Check sheet for the modelled part. Datum: model origin and axes. Units: mm. Face numbers are marked on the shaded views. A direction names the side the tool comes from. Coordinates: 2 decimals unless noted, no trailing zeros. Write each loop counter-clockwise with the first axis right and the second up, starting at its lowest first coordinate (ties: lowest second). Pieces come first, ordered by that corner, then holes. Notation, with made-up numbers: (1.5, 31.25) - (40.5, 31.25) arc R6 cw to (40.5, 39.25) - close; hole circle Ø1 at (78.25, 31). An arc over 180 degrees is marked (long way). Answer as CSV lines item,"result". Start each with the question number.
from build123d import *

# Parameters (mm, degrees)
BOSS_EXTRUDE1_DEPTH = 40
SKETCH2_R           = 4.25
CUT_EXTRUDE1_DEPTH  = 1


with BuildPart() as part:
    # Sketch1 → Boss-Extrude1 (new body)
    with BuildSketch(Plane.XY):
        Polygon((0, 0), (40, 0), (40, -1), (1, -1), (1, -51), (100, -51), (100, -52), (0, -52), align=None)
    extrude(amount=BOSS_EXTRUDE1_DEPTH)

    # Sketch2 → Cut-Extrude1 (cut)
    with BuildSketch(Plane.ZY):
        with Locations((20, -26)):
            Circle(SKETCH2_R)
    extrude(amount=-CUT_EXTRUDE1_DEPTH, mode=Mode.SUBTRACT)


solid = part.part
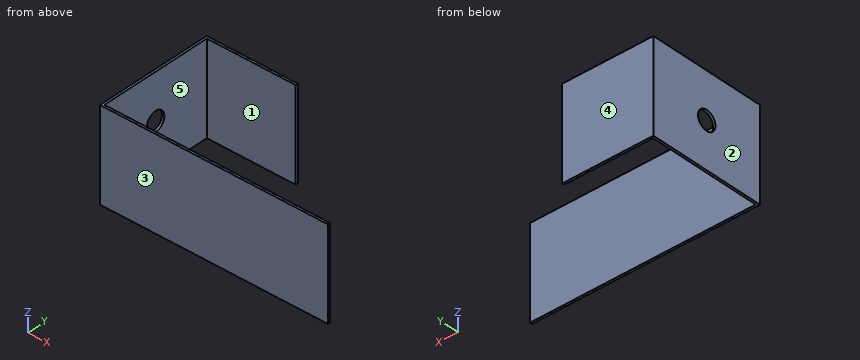
(1) Tool access check on the marked faces 4 and 5. Record the directions out of +Z, -Z, +X, -X, +Y, -Y that give a thin tool (end or side, any length) a straight path to the whole face; none if there is none.
(2) Material ranges on probe 1 along Y at (x, z) = (0.45, 20); probe 2 along Y at (x, z) = (12, 18.5); probe 3 along X at (y, z) = (-12, 18), recorded low to high. Write a range as from..to.
(3) Release check for a two-part mould opening along Y. For the marked faces 1, 2 and 3 record: pulls with the +Y half, pulls with the -Y half, needs draft (parallel to the pull), parting line crosses it, or undercut.
(4) Cross-section at B-B on z = 20. Record the boundary of the cut face in (x, y), plus the area to 4 significant figures.
(5) Cross-section at D-D on z = 29.5. Record the boundary of the cut face in (x, y).
(6) Cross-section at A-A on x = 17. Record the boundary of the cut face in (y, z), plus the area to 3 significant figures.
(7) Go/stop test with flat-tipped pins: P1, Ø12, axis at y = -37.5, z = 11, coming from the +X side; P2, Ø0.5, axis at y = -0.5, z = 17, coming from the +X side. Record where each tip stops, or that it passes through.
(8) Cross-section at C-C on y = -26. Record the boundary of the cut face in (x, z), plus the area to 3 significant figures.
Checked values:
1,face 4,"+Z, -Z, +X, -X, +Y"
1,face 5,"+Z, -Z, +X"
2,probe 1,"-52..-30.25, -21.75..0"
2,probe 2,"-52..-51, -1..0"
2,probe 3,"0..1"
3,face 1,"undercut"
3,face 2,"needs draft"
3,face 3,"pulls with the -Y half"
4,outline,"(0, -52) - (100, -52) - (100, -51) - (1, -51) - (1, -30.25) - (0, -30.25) - close; (0, -21.75) - (1, -21.75) - (1, -1) - (40, -1) - (40, 0) - (0, 0) - close"
4,area,"181.5 mm^2"
5,outline,"(0, -52) - (100, -52) - (100, -51) - (1, -51) - (1, -1) - (40, -1) - (40, 0) - (0, 0) - close"
6,outline,"(-52, 0) - (-51, 0) - (-51, 40) - (-52, 40) - close; (-1, 0) - (0, 0) - (0, 40) - (-1, 40) - close"
6,area,"80.0 mm^2"
7,P1,"x = 1"
7,P2,"x = 40"
8,outline,"(0, 0) - (1, 0) - (1, 15.75) - (0, 15.75) - close; (0, 24.25) - (1, 24.25) - (1, 40) - (0, 40) - close"
8,area,"31.5 mm^2"
